Could you check a few things on this model? Use its own coordinates, in mm. A direction names the side the tool comes from. Give positions to 0.01 mm unless a question says otherwise; leave off trailing zeros. Order: outer loops, then holes, each group sorted by start corner. A loop starts at its lowest first (then second) coordinate and runs counter-clockwise, first axis right, second up.
from build123d import *

# Parameters (mm, degrees)
SKETCH_1_W                      = 28
SKETCH_1_H                      = 60
SKETCH_1_R                      = 2.05
SKETCH_1_W_2                    = 20
SKETCH_1_H_2                    = 40.2
EXTRUDE_1_DEPTH                 = 28
CUT_EXTRUDE_3_DEPTH             = 51.714987923
CUT_EXTRUDE_3_DEPTH_BACK        = 51.714987923
SKETCH_4_W                      = 16
SKETCH_4_H                      = 22
FILLET_3_R                      = 5
FILLET_1_R                      = 3
SKETCH_6_R                      = 2.05
SKETCH_6_R_2                    = 1.6
EXTRUDE_3_DEPTH                 = 3
CUT_EXTRUDE_4_REACH             = 52.715
SKETCH_7_W                      = 9
SKETCH_7_H                      = 9.9
CUT_EXTRUDE_4_DIRECTION_2_DEPTH = 51.714987923
SKETCH_9_W                      = 20
SKETCH_9_H                      = 40.2
EXTRUDE_4_DEPTH                 = 1
FILLET_4_R                      = 0.5


with BuildPart() as part:
    # 草图1 → 凸台-拉伸1 (new body)
    with BuildSketch(Plane(origin=(0, 0, 0), x_dir=(1, 0, 0), z_dir=(0, 1, 0))):
        with Locations((0, -9.9)):
            Rectangle(SKETCH_1_W, SKETCH_1_H)
        with Locations(Location((-5, 14.1, 0), (0, 0, 270))):
            Circle(SKETCH_1_R, mode=Mode.SUBTRACT)
        with Locations(Location((5, 14.1, 0), (0, 0, 270))):
            Circle(SKETCH_1_R, mode=Mode.SUBTRACT)
        with Locations(Location((-5, -33.9, 0), (0, 0, 270))):
            Circle(SKETCH_1_R, mode=Mode.SUBTRACT)
        with Locations(Location((5, -33.9, 0), (0, 0, 270))):
            Circle(SKETCH_1_R, mode=Mode.SUBTRACT)
        with Locations((0, -9.9)):
            Rectangle(SKETCH_1_W_2, SKETCH_1_H_2, mode=Mode.SUBTRACT)
    extrude(amount=EXTRUDE_1_DEPTH)

    # 草图4 → 切除-拉伸3 (cut, two sides: drawn at the far end of the back side and taken through both)
    with BuildSketch(Plane(origin=(0, 0, 0), x_dir=(0, 0, -1), z_dir=(1, 0, 0)).offset(-CUT_EXTRUDE_3_DEPTH_BACK)):
        with Locations((-31.9, 14)):
            Rectangle(SKETCH_4_W, SKETCH_4_H)
        with BuildLine():
            Line((-12.9, 25), (5.1, 25))
            ThreePointArc((5.1, 25), (7.221320344, 24.121320344), (8.1, 22))
            Line((8.1, 22), (8.1, 6))
            ThreePointArc((8.1, 6), (7.221320344, 3.878679656), (5.1, 3))
            Line((5.1, 3), (-12.9, 3))
            ThreePointArc((-12.9, 3), (-15.021320344, 3.878679656), (-15.9, 6))
            Line((-15.9, 6), (-15.9, 22))
            ThreePointArc((-15.9, 22), (-15.021320344, 24.121320344), (-12.9, 25))
        make_face()
    extrude(amount=CUT_EXTRUDE_3_DEPTH + CUT_EXTRUDE_3_DEPTH_BACK, mode=Mode.SUBTRACT)

    # 圆角3
    fillet_3_edges = [part.edges().sort_by_distance(p)[0] for p in [
        (-12, 25, 23.9),
        (12, 25, 23.9),
        (12, 3, 23.9),
        (-12, 3, 23.9),
    ]]
    fillet(fillet_3_edges, radius=FILLET_3_R)

    # 圆角1
    fillet_1_edges = [part.edges().sort_by_distance(p)[0] for p in [
        (14, 1.5, 39.9),
        (-14, 1.5, 39.9),
        (14, 26.5, 39.9),
        (-14, 26.5, 39.9),
        (-14, 14, -20.1),
        (14, 14, -20.1),
    ]]
    fillet(fillet_1_edges, radius=FILLET_1_R)

    # 草图6 → 凸台-拉伸3 (add)
    # profile 1 of 2: a face of its own
    with BuildSketch(Plane.XZ):
        with Locations(Location((-5, 33.9, 0), (0, 0, 90))):
            Circle(SKETCH_6_R)
        with Locations(Location((-5, 33.9, 0), (0, 0, 270))):
            Circle(SKETCH_6_R_2, mode=Mode.SUBTRACT)
    # profile 2 of 2: a face of its own
    with BuildSketch(Plane.XZ):
        with Locations(Location((5, 33.9, 0), (0, 0, 90))):
            Circle(SKETCH_6_R)
        with Locations(Location((5, 33.9, 0), (0, 0, 270))):
            Circle(SKETCH_6_R_2, mode=Mode.SUBTRACT)
    extrude(amount=-EXTRUDE_3_DEPTH)

    # 草图7 → 切除-拉伸4 (cut, up to next)
    with BuildSketch(Plane(origin=(0, 28, 0), x_dir=(1, 0, 0), z_dir=(0, 1, 0)), mode=Mode.PRIVATE) as cut_extrude_4_sk1:
        with Locations((0, -34.95)):
            Rectangle(SKETCH_7_W, SKETCH_7_H)
    cut_extrude_4_tool1 = extrude(cut_extrude_4_sk1.sketch, amount=-CUT_EXTRUDE_4_REACH, mode=Mode.PRIVATE) & part.part
    add(cut_extrude_4_tool1.solids().sort_by_distance((0, 28, 34.95))[0], mode=Mode.SUBTRACT)

    # 草图7 → 切除-拉伸4 direction 2 (cut)
    with BuildSketch(Plane(origin=(0, 28, 0), x_dir=(1, 0, 0), z_dir=(0, 1, 0))):
        with Locations((0, -34.95)):
            Rectangle(SKETCH_7_W, SKETCH_7_H)
    extrude(amount=CUT_EXTRUDE_4_DIRECTION_2_DEPTH, mode=Mode.SUBTRACT)

    # 草图9 → 凸台-拉伸4 (add)
    with BuildSketch(Plane.XZ):
        with Locations((0, 9.9)):
            Rectangle(SKETCH_9_W, SKETCH_9_H)
    extrude(amount=-EXTRUDE_4_DEPTH)

    # 圆角4
    fillet_4_edges = [part.edges().sort_by_distance(p)[0] for p in [
        (-4.5, 26.5, 30),
        (-4.5, 26.5, 39.9),
        (4.5, 26.5, 39.9),
        (4.5, 26.5, 30),
    ]]
    fillet(fillet_4_edges, radius=FILLET_4_R)


solid = part.part
Item 1: Imagine slicing it at B-B on y = 16.75. List the corners of the cut face in (x, z) for me.
Findings:
outline: (-14, -17.1) arc R3 ccw to (-11, -20.1) - (11, -20.1) arc R3 ccw to (14, -17.1) - (14, -8.1) - (10, -8.1) - (10, -10.2) - (-10, -10.2) - (-10, -8.1) - (-14, -8.1) - close; (-14, 15.9) - (-10, 15.9) - (-10, 23.9) - (-14, 23.9) - close; (10, 15.9) - (14, 15.9) - (14, 23.9) - (10, 23.9) - close; hole circle Ø4.1 at (-5, -14.1); hole circle Ø4.1 at (5, -14.1)
Item 2: Imagine slicing it at A-A on z = -14.1. List the corners of the cut face in (x, y) for me, then the cut area to 3 significant figures.
Findings:
outline: (-14, 0) - (-7.05, 0) - (-7.05, 28) - (-14, 28) - close; (-2.95, 0) - (2.95, 0) - (2.95, 28) - (-2.95, 28) - close; (7.05, 0) - (14, 0) - (14, 28) - (7.05, 28) - close
area: 554 mm2
Item 3: Please list where these lines run through material, in increasing order: line 1 along X through (y, z) = (7, -14.1); line 2 along X through (y, z) = (2.25, 33.9); line 3 along Y through (x, z) = (-11.5, 4).
Findings:
line 1: x = -14 to -7.05, -2.95 to 2.95, 7.05 to 14
line 2: x = -14 to -6.6, -3.4 to 3.4, 6.6 to 14
line 3: y = 0 to 3, 25 to 28
Item 4: We'd pull the mould along X, two halves only. Please class faces 1 (the cylindrical face through (-4.93, 1.48, 35.5)), 2 (the cylindrical face through (-13.14, 26.52, 39)), 3 (the cylindrical face through (-12.03, 3.86, 15)): +X half, -X half, draft (parallel to the pull), parting line (faces both ways), or undercut.
Findings:
face 1: undercut
face 2: -X half
face 3: draft
Item 5: Imagine slicing it at C-C on z = 33.9. List the corners of the cut face in (x, y) for me.
Findings:
outline: (-14, 0) - (-6.6, 0) - (-6.6, 3) - (-14, 3) - close; (-14, 25) - (-7.05, 25) - (-7.05, 28) - (-14, 28) - close; (-3.4, 0) - (3.4, 0) - (3.4, 3) - (-3.4, 3) - close; (6.6, 0) - (14, 0) - (14, 3) - (6.6, 3) - close; (7.05, 25) - (14, 25) - (14, 28) - (7.05, 28) - close
Item 6: For pin 1 (2 mm diameter, centred on x = 5, z = -4.5, fed in from +Y); pin 2 (3 mm diameter, centred on x = 11, y = 10.5, fed in from +Z); pin 3 (3 mm diameter, centred on x = -5, z = 33.9, fed in from +Y); pin 4 (1.2 mm diameter, centred on x = 12.5, y = 13.5, fed in from -Z), each with a flat end and sliding along its axis, tell me the tip position at first contact or that it passes through.
Findings:
pin 1: stops at y = 1
pin 2: stops at z = 23.9
pin 3: passes through
pin 4: stops at z = -19.96
Item 7: For faces 4 (the flat face through (4.5, 27, 38)), 5 (the flat face through (-10, 14, 19)), 6 (the cylindrical face through (11.97, 3.9, -7.24)), 7 (the cylindrical face through (-13.14, 14.2, -19.2)), 8 (the flat face through (-9, 25, 34)), which set-ups out of +Z, -Z, +X, -X, +Y, -Y let a thin tool reach every point of the face, with its end or its side?
Findings:
face 4: +Z, +Y
face 5: +Y
face 6: +X, -X
face 7: -Z, -X, +Y, -Y
face 8: +Z, +X, -X
Item 8: Imagine slicing it at D-D on x = 6. List the corners of the cut face in (y, z) for me.
Findings:
outline: (0, -20.1) - (28, -20.1) - (28, -15.89) - (0, -15.89) - close; (0, -12.31) - (28, -12.31) - (28, -10.2) - (1, -10.2) - (1, 30) - (3, 30) - (3, 32.65) - (0, 32.65) - close; (0, 35.15) - (3, 35.15) - (3, 39.9) - (0, 39.9) - close; (25, 30) - (28, 30) - (28, 32.11) - (25, 32.11) - close; (25, 35.69) - (28, 35.69) - (28, 39.9) - (25, 39.9) - close
